The listing builds one solid part. Answer for the finished solid, in the listing's coordinates (mm). Round coordinates to 2 decimals unless told otherwise and drop trailing zeros. Write each loop counter-clockwise with the first axis right and the second up, starting at its lowest first coordinate (ties: lowest second). Pieces come first, ordered by that corner, then holes. Notation, with made-up numbers: (66.25, 40.5) - (95.25, 40.5) arc R27 ccw to (95.25, 77.5) - close; hole circle Ø11 at (-37.75, 72). An arc over 180 degrees is marked (long way). Return JSON: item names as keys, results as strings. Group by question number.
(1) Find the intervals of material crossed by line 1 along X through (y, z) = (0.7, 12.5); line 2 along X through (y, z) = (0.55, 12.5); line 3 along Z through (x, y) = (-15, 0.7), in increasing order. Write a range as [from, to].
(2) Section B-B, the plane x = -4.75 is taken. Write down the section's boundary in (y, z), then the cut area to 4 significant figures.
(3) Each of these flat-tipped pins is pushed along its axis until it touches: pin 1 (1.2 mm diameter, centred on x = 15.5, y = -1, fed in from -Z); pin 2 (2.5 mm diameter, centred on x = 15, z = 12.5, fed in from -Y); pin 3 (8 mm diameter, centred on x = -15, z = -12.5, fed in from -Y); pin 4 (1.2 mm diameter, centred on x = 16.5, y = -1, fed in from +Z). Where does it stop, or does it pass through?
(4) Section C-C, the plane z = -11.5 is taken. Write down the section's boundary in (x, y).
(5) Section D-D, the plane y = -1 is taken. Write down the section's boundary in (x, z), then the cut area to 3 significant figures.
(6) Section A-A, the plane z = 0 is taken. Write down the section's boundary in (x, y), then the cut area to 3 significant figures.
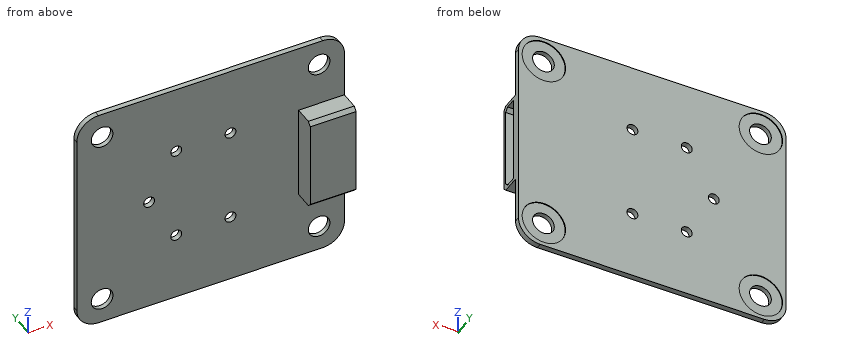
```python
from build123d import *

# Parameters (mm, degrees)
BOSS_EXTRUDE1_DEPTH = 0.75
CUT_EXTRUDE3_DEPTH  = 0.1
SKETCH3_R           = 1.5
CUT_EXTRUDE4_DEPTH  = 3.1
SKETCH4_R           = 0.75
CUT_EXTRUDE5_DEPTH  = 10
SKETCH6_W           = 6.340818297
SKETCH6_H           = 13.007496706
BOSS_EXTRUDE2_DEPTH = 3
SKETCH7_W           = 12.068220188
SKETCH7_H           = 2.061032276
CUT_EXTRUDE6_DEPTH  = 5
CHAMFER2_SIZE       = 0.5


with BuildPart() as part:
    # Sketch1 → Boss-Extrude1 (new body)
    with BuildSketch(Plane(origin=(0, 0, 0), x_dir=(1, 0, 0), z_dir=(0, 1, 0))):
        with BuildLine():
            Line((-15.5, 16), (15.5, 16))
            ThreePointArc((15.5, 16), (17.621320344, 15.121320344), (18.5, 13))
            Line((18.5, 13), (18.5, -13))
            ThreePointArc((18.5, -13), (17.621320344, -15.121320344), (15.5, -16))
            Line((15.5, -16), (-15.5, -16))
            ThreePointArc((-15.5, -16), (-17.621320344, -15.121320344), (-18.5, -13))
            Line((-18.5, -13), (-18.5, 13))
            ThreePointArc((-18.5, 13), (-17.621320344, 15.121320344), (-15.5, 16))
        make_face()
    extrude(amount=BOSS_EXTRUDE1_DEPTH)

    # Sketch2 → Cut-Extrude3 (cut)
    with BuildSketch(Plane(origin=(0, 0.75, 0), x_dir=(1, 0, 0), z_dir=(0, 1, 0))):
        with BuildLine():
            ThreePointArc((-15, 11), (-16.060660172, 13.560660172), (-13.5, 12.5))
            Line((-13.5, 12.5), (-12, 12.5))
            ThreePointArc((-12, 12.5), (-17.121320344, 14.621320344), (-15, 9.5))
            Line((-15, 9.5), (-15, 11))
        make_face()
        with BuildLine():
            Line((-12, 12.5), (-13.5, 12.5))
            ThreePointArc((-13.5, 12.5), (-13.939339828, 11.439339828), (-15, 11))
            Line((-15, 11), (-15, 9.5))
            ThreePointArc((-15, 9.5), (-12.878679656, 10.378679656), (-12, 12.5))
        make_face()
        with BuildLine():
            ThreePointArc((18, 12.5), (15, 15.5), (12, 12.5))
            Line((12, 12.5), (13.5, 12.5))
            ThreePointArc((13.5, 12.5), (15, 14), (16.5, 12.5))
            ThreePointArc((16.5, 12.5), (16.060660172, 11.439339828), (15, 11))
            Line((15, 11), (15, 9.5))
            ThreePointArc((15, 9.5), (17.121320344, 10.378679656), (18, 12.5))
        make_face()
        with BuildLine():
            Line((13.5, 12.5), (12, 12.5))
            ThreePointArc((12, 12.5), (12.878679656, 10.378679656), (15, 9.5))
            Line((15, 9.5), (15, 11))
            ThreePointArc((15, 11), (13.939339828, 11.439339828), (13.5, 12.5))
        make_face()
        with BuildLine():
            ThreePointArc((18, -12.5), (17.121320344, -10.378679656), (15, -9.5))
            Line((15, -9.5), (15, -11))
            ThreePointArc((15, -11), (16.060660172, -11.439339828), (16.5, -12.5))
            ThreePointArc((16.5, -12.5), (15, -14), (13.5, -12.5))
            Line((13.5, -12.5), (12, -12.5))
            ThreePointArc((12, -12.5), (15, -15.5), (18, -12.5))
        make_face()
        with BuildLine():
            Line((15, -11), (15, -9.5))
            ThreePointArc((15, -9.5), (12.878679656, -10.378679656), (12, -12.5))
            Line((12, -12.5), (13.5, -12.5))
            ThreePointArc((13.5, -12.5), (13.939339828, -11.439339828), (15, -11))
        make_face()
        with BuildLine():
            ThreePointArc((-12, -12.5), (-12.878679656, -10.378679656), (-15, -9.5))
            Line((-15, -9.5), (-15, -11))
            ThreePointArc((-15, -11), (-13.939339828, -11.439339828), (-13.5, -12.5))
            Line((-13.5, -12.5), (-12, -12.5))
        make_face()
        with BuildLine():
            Line((-15, -11), (-15, -9.5))
            ThreePointArc((-15, -9.5), (-17.121320344, -14.621320344), (-12, -12.5))
            Line((-12, -12.5), (-13.5, -12.5))
            ThreePointArc((-13.5, -12.5), (-16.060660172, -13.560660172), (-15, -11))
        make_face()
    extrude(amount=-CUT_EXTRUDE3_DEPTH, mode=Mode.SUBTRACT)

    # Sketch3 → Cut-Extrude4 (cut)
    with BuildSketch(Plane(origin=(0, 0.75, 0), x_dir=(1, 0, 0), z_dir=(0, 1, 0))):
        with Locations(Location((-15, 12.5, 0), (0, 0, 270))):
            Circle(SKETCH3_R)
        with Locations(Location((15, 12.5, 0), (0, 0, 270))):
            Circle(SKETCH3_R)
        with Locations(Location((-15, -12.5, 0), (0, 0, 270))):
            Circle(SKETCH3_R)
        with Locations(Location((15, -12.5, 0), (0, 0, 270))):
            Circle(SKETCH3_R)
    extrude(amount=-CUT_EXTRUDE4_DEPTH, mode=Mode.SUBTRACT)

    # Sketch4 → Cut-Extrude5 (cut)
    with BuildSketch(Plane(origin=(0, 0.75, 0), x_dir=(1, 0, 0), z_dir=(0, 1, 0))):
        with Locations(Location((2.75, -6.495190528, 0), (0, 0, 270))):
            Circle(SKETCH4_R)
        with Locations(Location((-4.75, -6.495190528, 0), (0, 0, 270))):
            Circle(SKETCH4_R)
        with Locations(Location((-8.5, 0, 0), (0, 0, 270))):
            Circle(SKETCH4_R)
        with Locations(Location((-4.75, 6.495190528, 0), (0, 0, 270))):
            Circle(SKETCH4_R)
        with Locations(Location((2.75, 6.495190528, 0), (0, 0, 270))):
            Circle(SKETCH4_R)
    extrude(amount=-CUT_EXTRUDE5_DEPTH, mode=Mode.SUBTRACT)

    # Sketch6 → Boss-Extrude2 (add)
    with BuildSketch(Plane.XZ):
        with Locations((15.329590852, 0)):
            Rectangle(SKETCH6_W, SKETCH6_H)
    extrude(amount=BOSS_EXTRUDE2_DEPTH)

    # Sketch7 → Cut-Extrude6 (cut)
    with BuildSketch(Plane(origin=(18.5, 0, 0), x_dir=(0, 0, -1), z_dir=(1, 0, 0))):
        with Locations((0, -1.5)):
            Rectangle(SKETCH7_W, SKETCH7_H)
    extrude(amount=-CUT_EXTRUDE6_DEPTH, mode=Mode.SUBTRACT)

    # Chamfer2
    chamfer2_edges = [part.edges().sort_by_distance(p)[0] for p in [
        (15.329590852, -3, -6.503748353),
        (15.329590852, -3, 6.503748353),
        (16, -2.530516138, 6.034110094),
        (16, -2.530516138, -6.034110094),
    ]]
    chamfer(chamfer2_edges, length=CHAMFER2_SIZE)


solid = part.part
```
Working result:
{
 "1": {"line 1": "x = [-18.5, -18], [-12, 12], [18, 18.5]", "line 2": "x = [-18.5, -16.5], [-13.5, 13.5], [16.5, 18.5]", "line 3": "z = [-16, -15.5], [-9.5, 9.5], [15.5, 16]"},
 "2": {"outline": "(0, -16) - (0.75, -16) - (0.75, -7.25) - (0, -7.25) - close; (0, -5.75) - (0.75, -5.75) - (0.75, 5.75) - (0, 5.75) - close; (0, 7.25) - (0.75, 7.25) - (0.75, 16) - (0, 16) - close", "area": "21.75 mm^2"},
 "3": {"pin 1": "stops at z = -6.5", "pin 2": "passes through", "pin 3": "stops at y = 0", "pin 4": "stops at z = 6.5"},
 "4": {"outline": "(-18.5, 0) - (-16.12, 0) - (-16.12, 0.65) - (-17.83, 0.65) - (-17.83, 0.75) - (-18.5, 0.75) - close; (-13.88, 0) - (13.88, 0) - (13.88, 0.65) - (12.17, 0.65) - (12.17, 0.75) - (-12.17, 0.75) - (-12.17, 0.65) - (-13.88, 0.65) - close; (16.12, 0) - (18.5, 0) - (18.5, 0.75) - (17.83, 0.75) - (17.83, 0.65) - (16.12, 0.65) - close"},
 "5": {"outline": "(12.16, -6.5) - (18.5, -6.5) - (18.5, -6.03) - (13.5, -6.03) - (13.5, 6.03) - (18.5, 6.03) - (18.5, 6.5) - (12.16, 6.5) - close", "area": "22.1 mm^2"},
 "6": {"outline": "(-18.5, 0) - (-9.25, 0) - (-9.25, 0.75) - (-18.5, 0.75) - close; (-7.75, 0) - (12.16, 0) - (12.16, -3) - (18.5, -3) - (18.5, -2.53) - (13.5, -2.53) - (13.5, -0.47) - (18.5, -0.47) - (18.5, 0.75) - (-7.75, 0.75) - close", "area": "35.3 mm^2"}
}
